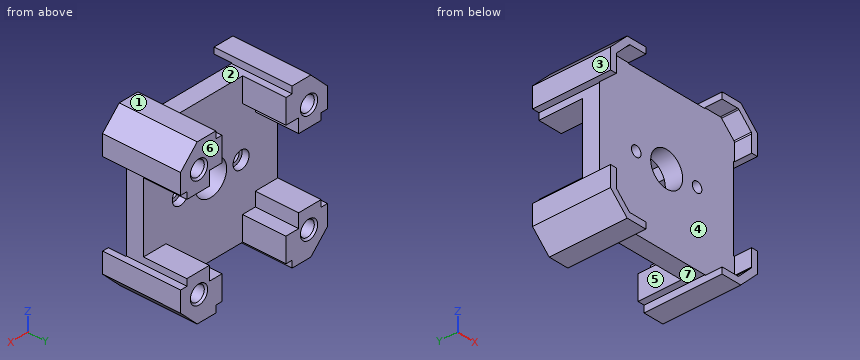
```python
from build123d import *

# Parameters (mm, degrees)
SKETCH1_R               = 1.5
SKETCH1_R_2             = 5
BOSS_EXTRUDE1_DEPTH     = 5
SKETCH2_W               = 28
SKETCH2_H               = 28
BOSS_EXTRUDE2_DEPTH     = 12.5
SKETCH3_R               = 2.2
CUT_EXTRUDE1_DEPTH      = 6
CUT_EXTRUDE2_DEPTH      = 62.921321045
CUT_EXTRUDE2_DEPTH_BACK = 62.921321045
SKETCH4_W               = 20
SKETCH4_H               = 23.078544061
CUT_EXTRUDE3_DEPTH      = 62.921321045
CUT_EXTRUDE3_DEPTH_BACK = 62.921321045
SKETCH5_W               = 20
SKETCH5_H               = 13.366359074
BOSS_EXTRUDE3_START     = -17.5
BOSS_EXTRUDE3_DEPTH     = 22.5
SKETCH8_R               = 2.5
CUT_EXTRUDE4_DEPTH      = 2
CUT_EXTRUDE5_DEPTH      = 5
FILLET1_R               = 0.5
CHAMFER1_SIZE           = 0.5


with BuildPart() as part:
    # Sketch1 → Boss-Extrude1 (new body)
    with BuildSketch(Plane(origin=(0, 0, 0), x_dir=(1, 0, 0), z_dir=(0, 1, 0))):
        Polygon((4.055, 0), (37.945, 0), (42, 4.055), (42, 37.945), (37.945, 42), (4.055, 42), (0, 37.945), (0, 4.055), align=None)
        with Locations(Location((11.475, 21, 0), (0, 0, 270))):
            Circle(SKETCH1_R, mode=Mode.SUBTRACT)
        with Locations(Location((30.525, 21, 0), (0, 0, 270))):
            Circle(SKETCH1_R, mode=Mode.SUBTRACT)
        with Locations(Location((21, 21, 0), (0, 0, 270))):
            Circle(SKETCH1_R_2, mode=Mode.SUBTRACT)
    extrude(amount=BOSS_EXTRUDE1_DEPTH)

    # Sketch2 → Boss-Extrude2 (add)
    with BuildSketch(Plane(origin=(0, 5, 0), x_dir=(1, 0, 0), z_dir=(0, 1, 0))):
        Polygon((37.945, 42), (4.055, 42), (0, 37.945), (0, 4.055), (4.055, 0), (37.945, 0), (42, 4.055), (42, 37.945), align=None)
        with Locations((21, 21)):
            Rectangle(SKETCH2_W, SKETCH2_H, mode=Mode.SUBTRACT)
    extrude(amount=BOSS_EXTRUDE2_DEPTH)

    # Sketch3 → Cut-Extrude1 (cut)
    with BuildSketch(Plane(origin=(0, 17.5, 0), x_dir=(1, 0, 0), z_dir=(0, 1, 0))):
        with Locations(Location((3.779747468, 36.775, 0), (0, 0, 270))):
            Circle(SKETCH3_R)
        with Locations(Location((3.779747468, 5.225, 0), (0, 0, 270))):
            Circle(SKETCH3_R)
        with Locations(Location((38.220252532, 5.225, 0), (0, 0, 90))):
            Circle(SKETCH3_R)
        with Locations(Location((38.220252532, 36.775, 0), (0, 0, 90))):
            Circle(SKETCH3_R)
    extrude(amount=-CUT_EXTRUDE1_DEPTH, mode=Mode.SUBTRACT)

    # Sketch4 → Cut-Extrude2 (cut, two sides: drawn at the far end of the back side and taken through both)
    with BuildSketch(Plane.ZY.offset(-CUT_EXTRUDE2_DEPTH_BACK)):
        with Locations((-21, 16.539272031)):
            Rectangle(SKETCH4_W, SKETCH4_H)
    extrude(amount=CUT_EXTRUDE2_DEPTH + CUT_EXTRUDE2_DEPTH_BACK, mode=Mode.SUBTRACT)

    # Sketch5 → Cut-Extrude3 (cut, two sides: drawn at the far end of the back side and taken through both)
    with BuildSketch(Plane(origin=(0, 0, -42), x_dir=(-1, 0, 0), z_dir=(0, 0, -1)).offset(-CUT_EXTRUDE3_DEPTH_BACK)):
        with Locations((-21, 11.683179537)):
            Rectangle(SKETCH5_W, SKETCH5_H)
    extrude(amount=CUT_EXTRUDE3_DEPTH + CUT_EXTRUDE3_DEPTH_BACK, mode=Mode.SUBTRACT)

    # Sketch7 → Boss-Extrude3 (add)
    with BuildSketch(Plane.XZ.offset(BOSS_EXTRUDE3_START)):
        Polygon((37.945, 0), (32.945, 0), (32.945, 2), (38.773427125, 2), (44, -3.226572875), (44, -9.055), (42, -9.055), (42, -4.055), align=None)
        Polygon((4.055, 0), (0, -4.055), (0, -9.055), (-2, -9.055), (-2, -3.226572875), (3.226572875, 2), (9.055, 2), (9.055, 0), align=None)
        Polygon((0, -37.945), (4.055, -42), (9.055, -42), (9.055, -44), (3.226572875, -44), (-2, -38.773427125), (-2, -32.945), (0, -32.945), align=None)
        Polygon((37.945, -42), (42, -37.945), (42, -32.945), (44, -32.945), (44, -38.773427125), (38.773427125, -44), (32.945, -44), (32.945, -42), align=None)
    extrude(amount=BOSS_EXTRUDE3_DEPTH)

    # Sketch8 → Cut-Extrude4 (cut)
    with BuildSketch(Plane(origin=(0, 5, 0), x_dir=(1, 0, 0), z_dir=(0, 1, 0))):
        with Locations(Location((11.475, 21, 0), (0, 0, 270))):
            Circle(SKETCH8_R)
        with Locations(Location((30.525, 21, 0), (0, 0, 270))):
            Circle(SKETCH8_R)
    extrude(amount=-CUT_EXTRUDE4_DEPTH, mode=Mode.SUBTRACT)

    # Sketch9 → Cut-Extrude5 (cut)
    with BuildSketch(Plane.XZ.offset(5)):
        Polygon((-0.2, -9.055), (-0.2, -3.972157288), (3.972157288, 0.2), (38.027842712, 0.2), (42.2, -3.972157288), (42.2, -38.027842712), (38.027842712, -42.2), (3.972157288, -42.2), (-0.2, -38.027842712), align=None)
    extrude(amount=-CUT_EXTRUDE5_DEPTH, mode=Mode.SUBTRACT)

    # Fillet1
    fillet1_edges = [part.edges().sort_by_distance(p)[0] for p in [
        (3.972157288, -2.5, 0.2),
        (-0.2, -2.5, -38.027842712),
        (-0.2, -2.5, -3.972157288),
        (38.027842712, -2.5, 0.2),
        (42.2, -2.5, -3.972157288),
        (42.2, -2.5, -38.027842712),
        (38.027842712, -2.5, -42.2),
        (3.972157288, -2.5, -42.2),
    ]]
    fillet(fillet1_edges, radius=FILLET1_R)

    # Chamfer1
    chamfer1_edges = [part.edges().sort_by_distance(p)[0] for p in [
        (38.220252532, 17.5, -34.575),
        (38.220252532, 17.5, -3.025),
        (3.779747468, 17.5, -7.425),
        (3.779747468, 17.5, -38.975),
    ]]
    chamfer(chamfer1_edges, length=CHAMFER1_SIZE)


solid = part.part
```
Work out the finished part from the listing and answer in its coordinate system (mm). Face numbers are marked on the shaded views. A direction names the side the tool comes from. Give positions to 0.01 mm unless a question says otherwise; leave off trailing zeros. Order: outer loops, then holes, each group sorted by start corner. A loop starts at its lowest first (then second) coordinate and runs counter-clockwise, first axis right, second up. Notation, with made-up numbers: (-5.75, -27) -> (7.25, -27) arc R18 ccw to (7.25, -18) -> close; hole circle Ø11 at (44, -4.75). An arc over 180 degrees is marked (long way). Answer as CSV lines item,"result". Start each with the question number.
(1) Section C-C, the plane y = 9.75 is taken. Give the number of separate pieces and of enclosed holes in the cut face, plus the area to 3 significant figures.
(2) Section D-D, the plane y = 0.75 is taken. Write down the section's boundary in (x, z) (3 decimals), plus the area to 3 significant figures.
(3) Which of the six approach directions +Z, -Z, +X, -X, +Y, -Y give full straight-line access (tool end or side, diameter ignored) to the marked faces 4, 5, 6 and 7?
(4) Consider line 1 along X through (y, z) = (2.2, -21) (3 decimals); line 2 along X through (y, z) = (-1.75, -35.5); line 3 along X through (y, z) = (12.75, -34). Determine where each line is inside the solid, lowest interval first.
(5) Each of these flat-tipped pins is pushed along its axis until it touches: pin 1 Ø5 at (x, z) = (3.78, -5.22) entering from +Y (3 decimals); pin 2 Ø7.5 at (x, y) = (3, 11) entering from +Z; pin 3 Ø2 at (y, z) = (7, -43) entering from -X; pin 4 Ø1.5 at (x, z) = (10, -20.5) entering from -Y. Where does it stop, or does it pass through?
(6) For a pull along X with two mould halves and no side action, classify the marked faces 1, 2 and 3 as released by +X, released by -X, zero draft, split by the parting line, or undercut.
(7) Section B-B, the plane z = -21 is taken. Write down the section's boundary in (x, y) (3 decimals), plus the area to 3 significant figures.
(8) Section A-A, the plane x = 21 is taken. Write down the section's boundary in (y, z), plus the area to 3 significant figures.
Entries:
1,separate pieces,"4"
1,enclosed holes,"0"
1,area,"526 mm²"
2,outline,"(-2, -38.773) -> (3.227, -44) -> (9.055, -44) -> (9.055, -42) -> (32.945, -42) -> (32.945, -44) -> (38.773, -44) -> (44, -38.773) -> (44, -32.945) -> (42, -32.945) -> (42, -9.055) -> (44, -9.055) -> (44, -3.227) -> (38.773, 2) -> (32.945, 2) -> (32.945, 0) -> (9.055, 0) -> (9.055, 2) -> (3.227, 2) -> (-2, -3.227) -> (-2, -9.055) -> (0, -9.055) -> (0, -32.945) -> (-2, -32.945) -> close; hole circle Ø3 at (11.475, -21); hole circle Ø10 at (21, -21); hole circle Ø3 at (30.525, -21)"
2,area,"1,780 mm²"
3,face 4,"-Y"
3,face 5,"+Z, -Z, +Y"
3,face 6,"+Z, -Z, +X, -X, +Y"
3,face 7,"-Z, +Y, -Y"
4,line 1,"0 to 9.975, 12.975 to 16, 26 to 29.025, 32.025 to 42"
4,line 2,"-2 to -0.2, 42.2 to 44"
4,line 3,"-2 to 7, 35 to 44"
5,pin 1,"y = 17.305"
5,pin 2,"z = 2"
5,pin 3,"x = 1.23"
5,pin 4,"y = 0"
6,face 1,"zero draft"
6,face 2,"undercut"
6,face 3,"released by -X"
7,outline,"(0, 0) -> (9.975, 0) -> (9.975, 3) -> (8.975, 3) -> (8.975, 5) -> (0, 5) -> close; (12.975, 0) -> (16, 0) -> (16, 5) -> (13.975, 5) -> (13.975, 3) -> (12.975, 3) -> close; (26, 0) -> (29.025, 0) -> (29.025, 3) -> (28.025, 3) -> (28.025, 5) -> (26, 5) -> close; (32.025, 0) -> (42, 0) -> (42, 5) -> (33.025, 5) -> (33.025, 3) -> (32.025, 3) -> close"
7,area,"122 mm²"
8,outline,"(0, -42) -> (5, -42) -> (5, -26) -> (0, -26) -> close; (0, -16) -> (5, -16) -> (5, 0) -> (0, 0) -> close"
8,area,"160 mm²"
